Here's how the part is built. I have some questions about the finished solid (model axes, mm). A direction names the side the tool comes from. Round coordinates to 2 decimals unless told otherwise and drop trailing zeros. Order: outer loops, then holes, each group sorted by start corner. A loop starts at its lowest first (then second) coordinate and runs counter-clockwise, first axis right, second up.
```python
from build123d import *

# Parameters (mm, degrees)
F1_DEPTH     = 5
F3_DEPTH     = 2
F4_T         = 2
F4_T4_ANGLE  = 97.3436104927
F4_T6_ANGLE  = 292.5225547035
F4_T8_ANGLE  = 97.3436104927
F4_T10_ANGLE = 262.1646662819
F5_R         = 2.5
F6_DEPTH     = 2


# Not quite as in the source:
# - a shell that OpenCascade refuses in one call is made with other operations: the cavity is built on its own and cut out


with BuildPart() as f1:
    # F0 (on Front) → F1 (new body)
    with BuildSketch(Plane.XZ):
        with BuildLine():
            ThreePointArc((31.5, 15), (30.3284271247, 17.8284271247), (27.5, 19))
            Line((27.5, 19), (-27.5, 19))
            ThreePointArc((-27.5, 19), (-30.3284271247, 17.8284271247), (-31.5, 15))
            Line((-31.5, 15), (-31.5, -15))
            ThreePointArc((-31.5, -15), (-30.3284271247, -17.8284271247), (-27.5, -19))
            Line((-27.5, -19), (27.5, -19))
            ThreePointArc((27.5, -19), (30.3284271247, -17.8284271247), (31.5, -15))
            Line((31.5, -15), (31.5, 15))
        make_face()
        with BuildLine():
            ThreePointArc((-1.6368421053, 9.4419116333), (29.5, 0), (-1.6368421053, -9.4419116333))
            ThreePointArc((-1.6368421053, -9.4419116333), (-3.0358514886, -8.5702451163), (-4.6142857143, -9.0451926571))
            ThreePointArc((-4.6142857143, -9.0451926571), (-24.5, 0), (-4.6142857143, 9.0451926571))
            ThreePointArc((-4.6142857143, 9.0451926571), (-3.0358514886, 8.5702451163), (-1.6368421053, 9.4419116333))
        make_face(mode=Mode.SUBTRACT)
    extrude(amount=F1_DEPTH)

    # F2 (on face) → F3 (join)
    with BuildSketch(Plane(origin=(0, 0, 0), x_dir=(-1, 0, 0), z_dir=(0, 1, 0))):
        with BuildLine():
            Line((27.5, 19), (-27.5, 19))
            ThreePointArc((-27.5, 19), (-30.3284271247, 17.8284271247), (-31.5, 15))
            Line((-31.5, 15), (-31.5, -15))
            ThreePointArc((-31.5, -15), (-30.3284271247, -17.8284271247), (-27.5, -19))
            Line((-27.5, -19), (27.5, -19))
            ThreePointArc((27.5, -19), (30.3284271247, -17.8284271247), (31.5, -15))
            Line((31.5, -15), (31.5, 15))
            ThreePointArc((31.5, 15), (30.3284271247, 17.8284271247), (27.5, 19))
        make_face()
    extrude(amount=F3_DEPTH)

    # F4: shell of thickness 2, made by hand


with BuildPart() as f4_core1:
    # F4_t2: copy of F1
    add(f1.part)

    # the walls: a layer under each face that stays
    f4_faces = [f4_core1.faces().sort_by_distance(p)[0] for p in [
        (30.3284271247, -1.5, 17.8284271247),
        (0, 2, 0),
        (-30.3284271247, -1.5, 17.8284271247),
        (-31.5, -1.5, 0),
        (-30.3284271247, -1.5, -17.8284271247),
        (0, -1.5, -19),
        (30.3284271247, -1.5, -17.8284271247),
        (0, -1.5, 19),
        (2.5, 0, 0),
        (29.5, -2.5, 0),
        (-24.5, -2.5, 0),
        (31.5, -1.5, 0),
    ]]
    thicken(f4_faces, amount=-F4_T, mode=Mode.SUBTRACT)

    # F4_s3 → F4_t4 (revolve, cut)
    with BuildSketch(Plane(origin=(3.8559556787, 0, -5.7733051009), x_dir=(0, 1, 0), z_dir=(0.5554065667, 0, -0.8315789474))):
        Polygon((-0.02, -6.5852631579), (0, -8.6052631579), (2, -8.6052631579), (2, -6.6052631579), align=None)
    revolve(axis=Axis((-3.3, 0, -10.5527247666), (0, -1, 0)), revolution_arc=F4_T4_ANGLE, mode=Mode.SUBTRACT)

    # F4_s5 → F4_t6 (revolve, cut)
    with BuildSketch(Plane(origin=(3.8559556787, 0, 5.7733051009), x_dir=(0, 1, 0), z_dir=(-0.5554065667, 0, -0.8315789474))):
        Polygon((-0.02, -6.5852631579), (2, -6.6052631579), (2, -8.6052631579), (0, -8.6052631579), align=None)
    revolve(axis=Axis((12.5, 0, 0), (0, 1, 0)), revolution_arc=F4_T6_ANGLE, mode=Mode.SUBTRACT)

    # F4_s7 → F4_t8 (revolve, cut)
    with BuildSketch(Plane(origin=(-7.1020408163, 0, 6.1916497355), x_dir=(0, 1, 0), z_dir=(-0.7537660548, 0, 0.6571428571))):
        Polygon((-0.02, -3.7657142857), (2, -3.7857142857), (2, -5.7857142857), (0, -5.7857142857), align=None)
    revolve(axis=Axis((-3.3, 0, 10.5527247666), (0, -1, 0)), revolution_arc=F4_T8_ANGLE, mode=Mode.SUBTRACT)

    # F4_s9 → F4_t10 (revolve, cut)
    with BuildSketch(Plane(origin=(-7.1020408163, 0, -6.1916497355), x_dir=(0, 1, 0), z_dir=(0.7537660548, 0, 0.6571428571))):
        Polygon((-0.02, -3.7657142857), (2, -3.7857142857), (2, -5.7857142857), (0, -5.7857142857), align=None)
    revolve(axis=Axis((-12.5, 0, 0), (0, 1, 0)), revolution_arc=F4_T10_ANGLE, mode=Mode.SUBTRACT)


with BuildPart() as f1_1:
    add(f1.part)

    # what is left inside the walls is the cavity
    f4_cavity = [f4_core1.part.solids().sort_by_distance(p)[0] for p in [
        (25.949171, -3.333333, 13.449171),
        (25.949171, -3.333333, -13.449171),
        (-21.12132, -0.02, -13.222222),
    ]]
    add(f4_cavity, mode=Mode.SUBTRACT)

    # F5 (on face) → F6 (cut, through all)
    with BuildSketch(Plane.XZ):
        with Locations((-12.5, 0)):
            Circle(F5_R)
        with Locations((12.5, 0)):
            Circle(F5_R)
    extrude(amount=-F6_DEPTH, mode=Mode.SUBTRACT)


solid = f1_1.part
```
1. I need wall thicknesses on probe 1 along X at (y, z) = (-1.1, 0); probe 2 along Z at (x, y) = (12.5, -1.2); probe 3 along Z at (x, y) = (12.5, 0.7). Which ranges of each line are inside material? Lowest first, please.
Evaluation:
probe 1: x = -31.5 to -29.5, -26.5 to -24.5, 29.5 to 31.5
probe 2: z = -19 to -17, 17 to 19
probe 3: z = -19 to -2.5, 2.5 to 19
2. I'm going to push flat-ended pins straight in: P1, Ø19, axis at x = -12.5, z = 0, coming from the +Y side; P2, Ø4, axis at x = 16, z = 11.5, coming from the -Y side. Where does each tip first touch, or does it pass through?
Evaluation:
P1: stops at y = 2
P2: stops at y = 0
3. If we section it at C-C, the plane y = -1.75: Write out the boundary of the cut face in (x, z), and give its area (3 significant figures).
Evaluation:
outline: (-31.5, -15) arc R4 ccw to (-27.5, -19) - (27.5, -19) arc R4 ccw to (31.5, -15) - (31.5, 15) arc R4 ccw to (27.5, 19) - (-27.5, 19) arc R4 ccw to (-31.5, 15) - close; hole (-29.5, -15) arc R2 ccw to (-27.5, -17) - (4.01, -17) arc R19 cw to (-3.3, -10.55) arc R14 cw (long way) to (-3.3, 10.55) arc R19 cw to (4.01, 17) - (-27.5, 17) arc R2 ccw to (-29.5, 15) - close; hole (-4.61, -9.05) arc R2 cw to (-1.64, -9.44) arc R17 ccw (long way) to (-1.64, 9.44) arc R2 cw to (-4.61, 9.05) arc R12 ccw (long way) to start; hole (20.99, -17) - (27.5, -17) arc R2 ccw to (29.5, -15) - (29.5, -8.49) arc R19 cw to start; hole (20.99, 17) arc R19 cw to (29.5, 8.49) - (29.5, 15) arc R2 ccw to (27.5, 17) - close
area: 619 mm2
4. If we section it at D-D, the plane x = 12.5: Write out the boundary of the cut face in (y, z).
Evaluation:
outline: (-5, -19) - (2, -19) - (2, -2.5) - (0, -2.5) - (0, -17) - (-5, -17) - close; (-5, 17) - (0, 17) - (0, 2.5) - (2, 2.5) - (2, 19) - (-5, 19) - close
5. If we section it at A-A, the plane x = -12.5: Write out the boundary of the cut face in (y, z).
Evaluation:
outline: (-5, -19) - (2, -19) - (2, -2.5) - (0, -2.5) - (0, -12) - (-5, -12) - (-5, -14) - (0, -14) - (0, -17) - (-5, -17) - close; (-5, 12) - (0, 12) - (0, 2.5) - (2, 2.5) - (2, 19) - (-5, 19) - (-5, 17) - (0, 17) - (0, 14) - (-5, 14) - close
6. If we section it at B-B, the plane z = 0: Write out the boundary of the cut face in (x, y), and give its area (3 significant figures).
Evaluation:
outline: (-31.5, -5) - (-29.5, -5) - (-29.5, 0) - (-26.5, 0) - (-26.5, -5) - (-24.5, -5) - (-24.5, 0) - (-15, 0) - (-15, 2) - (-31.5, 2) - close; (-10, 0) - (10, 0) - (10, 2) - (-10, 2) - close; (15, 0) - (29.5, 0) - (29.5, -5) - (31.5, -5) - (31.5, 2) - (15, 2) - close
area: 136 mm2
7. On a 3-axis mill with a long thin cutter (end or side, diameter ignored), from which of +Z, -Z, +X, -X, +Y, -Y can I reach the whole of each face in a straight line? I mean faces 4 (the cylindrical face through (30.359, -1.549, -17.797)), 5 (the flat face through (-29.5, -3, 0)). Say none if no direction works.
Evaluation:
face 4: -Z, +X, +Y, -Y
face 5: -Y
8. If we mould it in two halves opening along X, with no side actions, what happens to faces 1 (the cylindrical face through (-30.359, -1.549, 17.797)), 2 (the flat face through (-26.3, 0, 3.9)), 3 (the flat face through (-2, -5, 11))? For each: released by +X, released by -X, zero draft, split by the parting line, or undercut.
Evaluation:
face 1: released by -X
face 2: undercut
face 3: zero draft
